Can you work these out from the model? Positions are in its coordinate system, mm. A direction names the side the tool comes from. Round coordinates to 2 decimals unless told otherwise and drop trailing zeros. Write each loop counter-clockwise with the first axis right and the second up, starting at its lowest first coordinate (ties: lowest second). Pieces come first, ordered by that corner, then holes. Notation, with made-up numbers: (-35.75, 69.5) - (-11.75, 69.5) arc R25 ccw to (-11.75, 102.5) - close; hole circle Ø1 at (77, -23.5). An arc over 180 degrees is marked (long way). One line per item, written item: value. Start each with the question number.
(1) If I drill on L1, parallel to Y at x = 0, z = 9.85; L2, parallel to Y at x = 0, z = 4; L3, parallel to Z at x = 59, y = -40, over which ranges is the centre line in solid material (lowest first)? Write a range as from..to.
(2) I'm going to push flat-ended pins straight in: pin 1 Ø7 at (y, z) = (-27, 96.5) entering from +X; pin 2 Ø7.5 at (x, y) = (-56.5, -34) entering from +Z; pin 3 Ø3 at (y, z) = (31.5, 94.5) entering from +X; pin 4 Ø2 at (y, z) = (41, 42) entering from -X. Where does each tip first touch, or does it pass through?
(3) I want a section at C-C on y = 31.75. Give the number of separate pieces and of enclosed holes in the cut face, plus the area to 3 significant figures.
(4) I want a section at B-B on z = 60. List the corners of the cut face in (x, y) for me.
(5) Thinking about a two-plate mould opening in Y: for faces 4 (the face through (-70.98, -22.35, 12.58)), 5 (the face through (-52.432, -27.734, 10.321)), 6 (the face through (-3.4, 43.2, 38.1)), which applies, +Y half, -Y half, draft (parallel to the pull), parting line (faces both ways), or undercut?
(6) On a 3-axis mill with a long thin cutter (end or side, diameter ignored), from which of +Z, -Z, +X, -X, +Y, -Y can I reach the whole of each face in a straight line? I mean faces 1 (the face through (54, 29, 7.874)), 2 (the face through (10.795, -27, 96)), 3 (the face through (26, 2, 19.05)). Say none if no direction works.
from build123d import *

# Parameters (mm, degrees)
FRONT_FILLET_R               = 5.08
FRONT_CHAMFER_SIZE           = 1.905
BLOCK_SKETCH_W               = 21.59
BLOCK_SKETCH_H               = 93.159413511
BLOCK_CUT_DEPTH              = 13.335
CIRCULAR_SKETCH_R            = 2.5527
CIRCULAR_CUT_DEPTH           = 140.7
CIRCULAR_PATTERN_COUNT       = 6
OUTER_CIRCULAR_SKETCH_R      = 4.7625
OUTER_CIRCULAR_CUT_DEPTH     = 4.826
OUTER_CIRCULAR_PATTERN_COUNT = 6
F_1_4_20_TOPMOST_CUT_REACH   = 167.839
F_1_4_20_TOPMOST_CUT_BORE_R  = 2.5527


with BuildPart() as part:
    # Base Sketch → Base Revolve (revolve)
    with BuildSketch(Plane(origin=(0, 0, 0), x_dir=(0, 0, -1), z_dir=(1, 0, 0)), mode=Mode.PRIVATE) as base_revolve_sk:
        Polygon((0, 76.2), (-12.7, 76.2), (-12.7, 50.8), (-38.1, 50.8), (-38.1, 38.1), (-101.6, 38.1), (-101.6, 25.4), (-31.75, 25.4), (-31.75, 28.575), (-19.05, 28.575), (-19.05, 25.4), (0, 25.4), align=None)
    revolve(base_revolve_sk.sketch.rotate(Axis((0, 0, 0), (0, 0, 1)), 90), axis=Axis((0, 0, 0), (0, 0, 1)))

    # Front Fillet
    front_fillet_edges = [part.edges().sort_by_distance(p)[0] for p in [
        (38.1, 0, 38.1),
        (50.8, 0, 12.7),
    ]]
    fillet(front_fillet_edges, radius=FRONT_FILLET_R)

    # Front Chamfer
    front_chamfer_edges = [part.edges().sort_by_distance(p)[0] for p in [
        (38.1, 0, 101.6),
        (50.8, 0, 38.1),
        (76.2, 0, 12.7),
    ]]
    chamfer(front_chamfer_edges, length=FRONT_CHAMFER_SIZE)

    # Block Sketch → Block Cut (cut)
    with BuildSketch(Plane.XY.offset(104.14)):
        with Locations((0, 14.829706756)):
            Rectangle(BLOCK_SKETCH_W, BLOCK_SKETCH_H)
    extrude(amount=-BLOCK_CUT_DEPTH, mode=Mode.SUBTRACT)

    # Circular Sketch → Circular Cut (cut, through all)
    with BuildSketch(Plane.XY.offset(12.7)):
        with Locations((0, 63.5)):
            Circle(CIRCULAR_SKETCH_R)
    circular_cut = extrude(amount=-CIRCULAR_CUT_DEPTH, mode=Mode.SUBTRACT)

    # Circular Pattern: Circular Cut ×6 about axis
    circular_pattern_axis = Axis((0, 0, 0), (0, 0, 1))
    for i in range(1, CIRCULAR_PATTERN_COUNT):
        add(circular_cut.rotate(circular_pattern_axis, i * 360 / CIRCULAR_PATTERN_COUNT), mode=Mode.SUBTRACT)

    # Outer Circular Sketch → Outer Circular Cut (cut)
    with BuildSketch(Plane.XY.offset(12.7)):
        with Locations((0, 63.5)):
            Circle(OUTER_CIRCULAR_SKETCH_R)
    outer_circular_cut = extrude(amount=-OUTER_CIRCULAR_CUT_DEPTH, mode=Mode.SUBTRACT)

    # Outer Circular Pattern: Outer Circular Cut ×6 about axis
    outer_circular_pattern_axis = Axis((0, 0, 0), (0, 0, 1))
    for i in range(1, OUTER_CIRCULAR_PATTERN_COUNT):
        add(outer_circular_cut.rotate(outer_circular_pattern_axis, i * 360 / OUTER_CIRCULAR_PATTERN_COUNT), mode=Mode.SUBTRACT)

    # 1/4-20 Topmost Cut bore (on position points) → 1/4-20 Topmost Cut (cut, up to next)
    with BuildSketch(Plane(origin=(0, 50.8, 26.9875), x_dir=(1, 0, 0), z_dir=(0, 1, 0)), mode=Mode.PRIVATE) as f_1_4_20_topmost_cut_sk1:
        Circle(F_1_4_20_TOPMOST_CUT_BORE_R)
    f_1_4_20_topmost_cut_tool1 = extrude(f_1_4_20_topmost_cut_sk1.sketch, amount=-F_1_4_20_TOPMOST_CUT_REACH, mode=Mode.PRIVATE) & part.part
    add(f_1_4_20_topmost_cut_tool1.solids().sort_by_distance((0, 50.8, 26.9875))[0], mode=Mode.SUBTRACT)


solid = part.part
Established:
1. L1: -76.2..-68.26, -58.74..-25.4, 25.4..58.74, 68.26..76.2
1. L2: -76.2..-66.05, -60.95..-25.4, 25.4..60.95, 66.05..76.2
1. L3: 0..12.7
2. pin 1: x = 29.99
2. pin 2: z = 12.7
2. pin 3: x = 23.49
2. pin 4: through
3. separate pieces: 3
3. enclosed holes: 1
3. area: 6,040 mm2
4. outline: circle Ø76.2 at (0, 0); hole circle Ø50.8 at (0, 0)
5. face 4: parting line
5. face 5: undercut
5. face 6: draft
6. face 1: +Z
6. face 2: +Z, +Y
6. face 3: none
